```python
from build123d import *

# Parameters (mm, degrees)
F0_W     = 46.9392
F0_H     = 158.48838
F1_DEPTH = 38.00094
F2_T     = -1.2192
F3_R     = 2.54
F5_DEPTH = 46.9402
F6_R     = 3.175
F7_DEPTH = 46.9402
F8_W     = 44.5008
F8_H     = 35.46094
F9_DEPTH = 1.2192


with BuildPart() as f1:
    # F0 (on Top) → F1 (new body)
    with BuildSketch(Plane.XY):
        Rectangle(F0_W, F0_H)
    extrude(amount=-F1_DEPTH)

    # F2
    f2_openings = [f1.faces().sort_by_distance(p)[0] for p in [
        (0, 0, -38.00094),
    ]]
    offset(amount=F2_T, openings=f2_openings)

    # F3
    f3_edges = [f1.edges().sort_by_distance(p)[0] for p in [
        (23.4696, 0, 0),
        (-23.4696, 0, 0),
        (0, -79.24419, 0),
        (23.4696, -79.24419, -19.00047),
        (-23.4696, -79.24419, -19.00047),
        (-23.4696, 79.24419, -19.00047),
        (23.4696, 79.24419, -19.00047),
        (0, 79.24419, 0),
    ]]
    fillet(f3_edges, radius=F3_R)

    # F4 (on face) → F5 (cut, through all)
    with BuildSketch(Plane.YZ.offset(23.4696)):
        with BuildLine():
            Line((4.74345, -38.00094), (34.74339, -38.00094))
            Line((34.74339, -38.00094), (34.74339, -31.00197))
            ThreePointArc((34.74339, -31.00197), (33.278927, -27.466443), (29.7434, -26.00198))
            Line((29.7434, -26.00198), (9.74344, -26.00198))
            ThreePointArc((9.74344, -26.00198), (6.207913, -27.466443), (4.74345, -31.00197))
            Line((4.74345, -31.00197), (4.74345, -38.00094))
        make_face()
    extrude(amount=-F5_DEPTH, mode=Mode.SUBTRACT)

    # F6 (on face) → F7 (cut, through all)
    with BuildSketch(Plane.YZ.offset(23.4696)):
        with Locations((-26.84399, -26.86304)):
            Circle(F6_R)
        with Locations((49.35601, -26.86304)):
            Circle(F6_R)
    extrude(amount=-F7_DEPTH, mode=Mode.SUBTRACT)

    # F8 (on face) → F9 (cut, through all)
    with BuildSketch(Plane(origin=(0, 79.24419, 0), x_dir=(-1, 0, 0), z_dir=(0, 1, 0))):
        with Locations((0, -20.27047)):
            Rectangle(F8_W, F8_H)
    extrude(amount=-F9_DEPTH, mode=Mode.SUBTRACT)


solid = f1.part
```
Geometry: final body of the model. Coordinates: model frame, mm. A direction names the side the tool comes from. Give positions to 0.01 mm unless a question says otherwise; leave off trailing zeros. Loops run counter-clockwise (first coordinate to the right, second up) from the corner with the lowest first, then second, coordinate; pieces in that order, holes last. Notation, with made-up numbers: (7.5, 13) - (18.5, 13) arc R36 ccw to (18.5, 51) - close; hole circle Ø4 at (21.5, 41). An arc over 180 degrees is marked (long way). Answer as CSV lines item,"result". Start each with the question number.
(1) Mould query, pull axis Z, two halves, no side actions, for faces 1 (the face through (-22.85, 33.32, -27.51)), 2 (the face through (22.869, 48.668, -29.963)), 3 (the face through (0, -79.244, -20)). Classes: +Z half, -Z half, draft (parallel to the pull), parting line (faces both ways), or undercut.
(2) Section query C-C (y = -35). Output: boundary loops of the cut face in (x, z), and give its area (3 significant figures).
(3) Ray query, line 1 along X through (y, z) = (71.5, -26.5); line 2 along Y through (x, z) = (14, -35.5); line 3 along Z through (x, y) = (-16, -47). Return the intervals inside material, ascending. Write a range as [from, to].
(4) Reachability of faces 4 (the face through (-22.851, 6.247, -27.428)), 5 (the face through (0, 1, 0)), 6 (the face through (0, 1, -1.219)) from +Z, -Z, +X, -X, +Y, -Y: full face, straight path, thin tool, end or side. Return the list, or none.
(5) Section query B-B (x = 18.5). Output: boundary loops of the cut face in (y, z).
(6) Pin query (flat end, axial travel): P1, Ø11, axis at x = -6, z = -20, coming from the +Y side (3 decimals); P2, Ø1.3, axis at x = 22.5, y = 16.5, coming from the -Z side; P3, Ø1.5, axis at x = 1, z = -1.5, coming from the -Y side. Return the tip coordinate at first contact, or that it passes through.
(7) Section query A-A (z = -8). Output: boundary loops of the cut face in (x, y).
Worked answers:
1,face 1,"-Z half"
1,face 2,"undercut"
1,face 3,"draft"
2,outline,"(-23.47, -38) - (-22.25, -38) - (-22.25, -1.22) - (22.25, -1.22) - (22.25, -38) - (23.47, -38) - (23.47, -2.54) arc R2.54 ccw to (20.93, 0) - (-20.93, 0) arc R2.54 ccw to (-23.47, -2.54) - close"
2,area,"144 mm^2"
3,line 1,"x = [-23.47, -22.25], [22.25, 23.47]"
3,line 2,"y = [-79.24, -78.02]"
3,line 3,"z = [-1.22, 0]"
4,face 4,"-Z, +X, -X"
4,face 5,"+Z, +X, -X, +Y, -Y"
4,face 6,"-Z"
5,outline,"(-79.24, -38) - (-78.02, -38) - (-78.02, -1.22) - (78.02, -1.22) - (78.02, -2.54) - (79.24, -2.54) arc R2.54 ccw to (76.7, 0) - (-76.7, 0) arc R2.54 ccw to (-79.24, -2.54) - close"
6,P1,"stops at y = -78.025"
6,P2,"stops at z = -26"
6,P3,"stops at y = -79.23"
7,outline,"(-23.47, -76.7) arc R2.54 ccw to (-20.93, -79.24) - (20.93, -79.24) arc R2.54 ccw to (23.47, -76.7) - (23.47, 76.7) arc R2.54 ccw to (22.25, 78.87) - (22.25, -78.02) - (-22.25, -78.02) - (-22.25, 78.87) arc R2.54 ccw to (-23.47, 76.7) - close"
